```python
from build123d import *

# Parameters (mm, degrees)
F0_W     = 124.53489
F0_H     = 53.96512
F1_DEPTH = 75
F4_R     = 7.882332
F3_R     = 8
F2_R     = 7.71025
F5_DEPTH = 50


with BuildPart() as f1:
    # F0 (on Front) → F1 (new body)
    with BuildSketch(Plane.XZ):
        with Locations((0, -0.244186)):
            Rectangle(F0_W, F0_H)
    extrude(amount=F1_DEPTH)

    # F4 (on face) + F3 (on face) + F2 (on face) → F5 (cut)
    with BuildSketch(Plane.XY.offset(26.738374)):
        with Locations((-48.593026, -58.238372)):
            Circle(F4_R)
        with Locations((-23.593026, -58.238372)):
            Circle(F4_R)
        with Locations((1.406974, -58.238372)):
            Circle(F4_R)
        with Locations((26.406974, -58.238372)):
            Circle(F4_R)
        with Locations((51.406974, -58.238372)):
            Circle(F4_R)
    with BuildSketch(Plane.XY.offset(26.738374)):
        with Locations((-47.880299, -34.304835)):
            Circle(F3_R)
        with Locations((-24.080299, -34.304835)):
            Circle(F3_R)
        with Locations((-0.280299, -34.304835)):
            Circle(F3_R)
        with Locations((23.519701, -34.304835)):
            Circle(F3_R)
        with Locations((47.319701, -34.304835)):
            Circle(F3_R)
    with BuildSketch(Plane.XY.offset(26.738374)):
        with Locations((-48.34884, -9.889536)):
            Circle(F2_R)
        with Locations((-24.54884, -9.889536)):
            Circle(F2_R)
        with Locations((-0.74884, -9.889536)):
            Circle(F2_R)
        with Locations((23.05116, -9.889536)):
            Circle(F2_R)
        with Locations((46.85116, -9.889536)):
            Circle(F2_R)
    extrude(amount=-F5_DEPTH, mode=Mode.SUBTRACT)


solid = f1.part
```
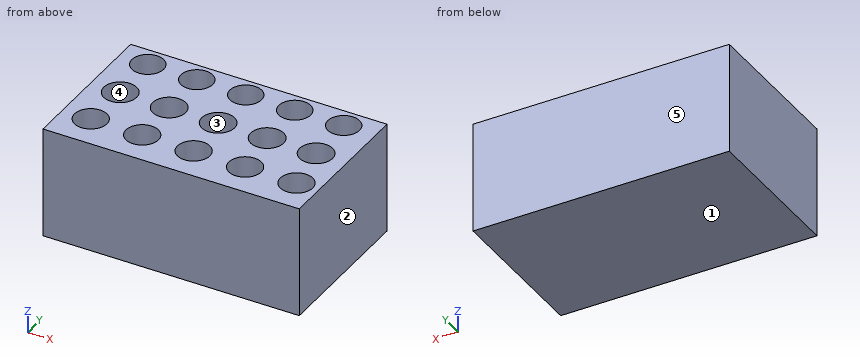
Build history of the part. All positions in model axes, mm. Face numbers are marked on the shaded views. A direction names the side the tool comes from. Round coordinates to 2 decimals unless told otherwise and drop trailing zeros. Write each loop counter-clockwise with the first axis right and the second up, starting at its lowest first coordinate (ties: lowest second). Pieces come first, ordered by that corner, then holes.
1) Drill centre lines: probe 1 along X at (y, z) = (-58, 24); probe 2 along Y at (x, z) = (-2, 5.5); probe 3 along Y at (x, z) = (48, 13). Where is each one in solid material? Low to high.
2) Band-saw the part on D-D, the plane x = -19.5. List the corners of the cut face in (y, z).
3) Band-saw the part on B-B, the plane y = -31. List the corners of the cut face in (x, z), and give its area (3 significant figures).
4) Band-saw the part on A-A, the plane z = -12. Give the number of separate pieces and of enclosed holes in the cut face, and give its area (3 significant figures).
5) 3-axis set-ups, long thin cutter, end or side, ignore diameter. For the marked faces 4 and 5: which of +Z, -Z, +X, -X, +Y, -Y reach the whole face in a straight line?
6) Pin check, flat tip, straight feed: pin 1 (5 mm diameter, centred on x = 43.5, y = -30.5, fed in from +Z). Stop position of the tip, or through.
7) Band-saw the part on C-C, the plane x = 48. List the corners of the cut face in (y, z).
8) Mould opens along X. For the marked faces 1, 2 and 3 say: +X half, -X half, draft (parallel to the pull), parting line (faces both ways), or undercut.
Ans:
1. probe 1: x = -62.27 to -56.47, -40.71 to -31.47, -15.71 to -6.47, 9.29 to 18.53, 34.29 to 43.53, 59.29 to 62.27
1. probe 2: y = -75 to -65.35, -51.13 to -42.12, -26.49 to -17.5, -2.28 to 0
1. probe 3: y = -75 to -65.35, -51.13 to -42.28, -26.33 to -17.51, -2.27 to 0
2. outline: (-75, -27.23) - (0, -27.23) - (0, 26.74) - (-4.06, 26.74) - (-4.06, -23.26) - (-15.72, -23.26) - (-15.72, 26.74) - (-27.75, 26.74) - (-27.75, -23.26) - (-40.86, -23.26) - (-40.86, 26.74) - (-51.5, 26.74) - (-51.5, -23.26) - (-64.97, -23.26) - (-64.97, 26.74) - (-75, 26.74) - close
3. outline: (-62.27, -27.23) - (62.27, -27.23) - (62.27, 26.74) - (54.61, 26.74) - (54.61, -23.26) - (40.03, -23.26) - (40.03, 26.74) - (30.81, 26.74) - (30.81, -23.26) - (16.23, -23.26) - (16.23, 26.74) - (7.01, 26.74) - (7.01, -23.26) - (-7.57, -23.26) - (-7.57, 26.74) - (-16.79, 26.74) - (-16.79, -23.26) - (-31.37, -23.26) - (-31.37, 26.74) - (-40.59, 26.74) - (-40.59, -23.26) - (-55.17, -23.26) - (-55.17, 26.74) - (-62.27, 26.74) - close
3. area: 3,080 mm2
4. separate pieces: 1
4. enclosed holes: 15
4. area: 6,430 mm2
5. face 4: +Z
5. face 5: +Z, -Z, +X, -X, +Y
6. pin 1: stops at z = -23.26
7. outline: (-75, -27.23) - (0, -27.23) - (0, 26.74) - (-2.27, 26.74) - (-2.27, -23.26) - (-17.51, -23.26) - (-17.51, 26.74) - (-26.33, 26.74) - (-26.33, -23.26) - (-42.28, -23.26) - (-42.28, 26.74) - (-51.13, 26.74) - (-51.13, -23.26) - (-65.35, -23.26) - (-65.35, 26.74) - (-75, 26.74) - close
8. face 1: draft
8. face 2: +X half
8. face 3: undercut
